```python
from build123d import *

# Parameters (mm, degrees)
SKETCH_R              = 17
PAD_DEPTH             = 30
SKETCH001_R           = 14
POCKET_DEPTH          = 20
SKETCH002_R           = 5
PAD001_DEPTH          = 2
SKETCH003_R           = 4
PAD002_DEPTH          = 9
FILLET_R              = 1
SKETCH004_W           = 47.033489
SKETCH004_H           = 47.446069
PAD003_DEPTH          = 10
SKETCH005_W           = 5.5
SKETCH005_H           = 5.5
POCKET001_DEPTH       = 15
POLARPATTERN_COUNT    = 3
SKETCH006_W           = 48.40057
SKETCH006_H           = 10.44081
POCKET002_DEPTH       = 47.447069
SKETCH007_W           = 6
SKETCH007_H           = 1.5
POCKET003_DEPTH       = 8
SKETCH008_R           = 0.776248
POCKET004_DEPTH       = 5
POLARPATTERN001_COUNT = 3
FILLET001_R           = 1


with BuildPart() as part:
    # Sketch → Pad (new body)
    with BuildSketch(Plane.XY):
        Circle(SKETCH_R)
    extrude(amount=PAD_DEPTH)

    # Sketch001 (on Face3 of Pad) → Pocket (cut)
    with BuildSketch(Plane.XY.offset(30)):
        Circle(SKETCH001_R)
    extrude(amount=-POCKET_DEPTH, mode=Mode.SUBTRACT)

    # Sketch002 (on Face5 of Pocket) → Pad001 (join)
    with BuildSketch(Plane.XY.offset(10)):
        Circle(SKETCH002_R)
    extrude(amount=PAD001_DEPTH)

    # Sketch003 (on Face7 of Pad001) → Pad002 (join)
    with BuildSketch(Plane.XY.offset(12)):
        Circle(SKETCH003_R)
    extrude(amount=PAD002_DEPTH)

    # Fillet
    fillet_edges = [part.edges().sort_by_distance(p)[0] for p in [
        (-4, 0, 21),
    ]]
    fillet(fillet_edges, radius=FILLET_R)

    # Sketch004 (on Face8 of Fillet) → Pad003 (join)
    with BuildSketch(Plane.XY.offset(30)):
        with Locations((0.145404, -0.183003)):
            Rectangle(SKETCH004_W, SKETCH004_H)
    extrude(amount=PAD003_DEPTH)

    # Sketch005 (on Face6 of Pad003) → Pocket001 (cut)
    with BuildSketch(Plane.XZ.offset(23.906038)):
        with Locations((0, 4.110798)):
            Rectangle(SKETCH005_W, SKETCH005_H)
    pocket001 = extrude(amount=-POCKET001_DEPTH, mode=Mode.SUBTRACT)

    # PolarPattern: Pocket001 ×3 about axis
    polarpattern_axis = Axis((0, 0, 0), (0, 0, 1))
    for i in range(1, POLARPATTERN_COUNT):
        add(pocket001.rotate(polarpattern_axis, i * 360 / POLARPATTERN_COUNT), mode=Mode.SUBTRACT)

    # Sketch006 (on Face6 of PolarPattern) → Pocket002 (cut, through all)
    with BuildSketch(Plane.XZ.offset(23.906038)):
        with Locations((0.264744, 35.122468)):
            Rectangle(SKETCH006_W, SKETCH006_H)
    extrude(amount=-POCKET002_DEPTH, mode=Mode.SUBTRACT)

    # Sketch007 (on Face2 of Pocket002) → Pocket003 (cut)
    with BuildSketch(Plane.XY.offset(29.902063)):
        with Locations((0.040436, 15.031708)):
            Rectangle(SKETCH007_W, SKETCH007_H)
    extrude(amount=-POCKET003_DEPTH, mode=Mode.SUBTRACT)

    # Sketch008 (on Face3 of Pocket003) → Pocket004 (cut)
    with BuildSketch(Plane(origin=(0, 0, 0), x_dir=(1, 0, 0), z_dir=(0, 0, -1))):
        with Locations((0, 15.325977)):
            Circle(SKETCH008_R)
    pocket004 = extrude(amount=-POCKET004_DEPTH, mode=Mode.SUBTRACT)

    # PolarPattern001: Pocket004 ×3 about axis
    polarpattern001_axis = Axis((0, 0, 0), (0, 0, -1))
    for i in range(1, POLARPATTERN001_COUNT):
        add(pocket004.rotate(polarpattern001_axis, i * 360 / POLARPATTERN001_COUNT), mode=Mode.SUBTRACT)

    # Fillet001
    fillet001_edges = [part.edges().sort_by_distance(p)[0] for p in [
        (-17, 0, 29.902063),
    ]]
    fillet(fillet001_edges, radius=FILLET001_R)


solid = part.part
```
Check sheet for the modelled part. Datum: model origin and axes. Units: mm. A direction names the side the tool comes from. Round coordinates to 2 decimals unless told otherwise and drop trailing zeros. Order: outer loops, then holes, each group sorted by start corner. A loop starts at its lowest first (then second) coordinate and runs counter-clockwise, first axis right, second up. Notation, with made-up numbers: (12.5, -30) -> (21.5, -30) arc R29 ccw to (21.5, 8) -> close; hole circle Ø4 at (13, 2.5). An arc over 180 degrees is marked (long way). One line per item, written item: value. Start each with the question number.
Q1. Cross-section at D-D (z = 24). Record the boundary of the cut face in (x, y).
Q2. Set-up check for faces 5 (the face through (0, -13, 1.361)), 6 (the face through (0, 0, 21)), 7 (the face through (12.543, 4.067, 4.072)), 8 (the face through (-0.17, -14.57, 0.67)): record each of +Z, -Z, +X, -X, +Y, -Y from which the full face is reachable in a straight line by a thin tool's end or side.
Q3. Thickness scan on line 1 (Z direction, x = 2, y = -13); line 2 (X direction, y = 0.5, z = 15.25); line 3 (Z direction, x = -4, y = 9). Record the ranges inside material, lowest first.
Q4. Cross-section at C-C (z = 2.5). Record the boundary of the cut face in (x, y), and give its area (3 significant figures).
Q5. Mould release check, pull along Z, two halves, no side actions. Record for faces 1 (the face through (1.1, -14.3, 29.902)), 2 (the face through (3.04, 15, 26)), 3 (the face through (-9.793, 8.83, 4.072)), 4 (the face through (7.73, 4.42, 4.15)): pulls with the +Z half, pulls with the -Z half, needs draft (parallel to the pull), parting line crosses it, or undercut.
Q6. Gauge pin test, flat ends, axial feed: pin 1 Ø6 at (x, z) = (-8, 16.5) entering from -Y; pin 2 Ø3 at (y, z) = (-6, 13.5) entering from +X; pin 3 Ø3 at (x, z) = (1, 3) entering from -Y. Record the tip position at first contact, or that the pin passes through.
Q7. Cross-section at B-B (y = 0). Record the boundary of the cut face in (x, z).
Completed:
1. outline: circle Ø34 at (0, 0); hole circle Ø28 at (0, 0); hole (-2.96, 14.28) -> (3.04, 14.28) -> (3.04, 15.78) -> (-2.96, 15.78) -> close
2. face 5: -Y
2. face 6: +Z
2. face 7: none
2. face 8: -Z
3. line 1: z = 0 to 1.36, 6.86 to 10
3. line 2: x = -16.99 to -13.99, -3.97 to 3.97, 13.99 to 16.99
3. line 3: z = 0 to 10
4. outline: (-15.9, 6.01) arc R17 ccw to (-2.75, -16.78) -> (-2.75, -8.91) -> (2.75, -8.91) -> (2.75, -16.78) arc R17 ccw to (15.9, 6.01) -> (9.09, 2.07) -> (6.34, 6.83) -> (13.15, 10.77) arc R17 ccw to (-13.15, 10.77) -> (-6.34, 6.83) -> (-9.09, 2.07) -> close
4. area: 776 mm²
5. face 1: pulls with the +Z half
5. face 2: needs draft
5. face 3: undercut
5. face 4: undercut
6. pin 1: stops at y = -16.25
6. pin 2: stops at x = 16.39
6. pin 3: stops at y = -8.91
7. outline: (-17, 0) -> (17, 0) -> (17, 28.9) arc R1 ccw to (16, 29.9) -> (14, 29.9) -> (14, 10) -> (5, 10) -> (5, 12) -> (4, 12) -> (4, 20) arc R1 ccw to (3, 21) -> (-3, 21) arc R1 ccw to (-4, 20) -> (-4, 12) -> (-5, 12) -> (-5, 10) -> (-14, 10) -> (-14, 29.9) -> (-16, 29.9) arc R1 ccw to (-17, 28.9) -> close
